```python
from build123d import *

# Parameters (mm, degrees)
SKETCH_1_R      = 25
EXTRUDE_1_DEPTH = 1
FILLET_1_R      = 1.6
EXTRUDE_START   = 5
EXTRUDE_3_DEPTH = 5
CHAMFER_3_SIZE  = 0.2


with BuildPart() as part:
    # 草图1 → 凸台-拉伸1 (new body)
    with BuildSketch(Plane.XY):
        Circle(SKETCH_1_R)
        with BuildLine():
            Line((-2.5, 1.658312395), (2.5, 1.658312395))
            ThreePointArc((2.5, 1.658312395), (0, -3), (-2.5, 1.658312395))
        make_face(mode=Mode.SUBTRACT)
        with BuildLine():
            ThreePointArc((-12.124355653, -7), (-7, -12.124355653), (0, -14))
            Line((0, -14), (0, -21))
            ThreePointArc((0, -21), (-10.5, -18.186533479), (-18.186533479, -10.5))
            Line((-18.186533479, -10.5), (-12.124355653, -7))
        make_face(mode=Mode.SUBTRACT)
        with BuildLine():
            ThreePointArc((0, 14), (-7, 12.124355653), (-12.124355653, 7))
            Line((-12.124355653, 7), (-18.186533479, 10.5))
            ThreePointArc((-18.186533479, 10.5), (-10.5, 18.186533479), (0, 21))
            Line((0, 21), (0, 14))
        make_face(mode=Mode.SUBTRACT)
        with BuildLine():
            Line((18.186533479, -10.5), (12.124355653, -7))
            ThreePointArc((12.124355653, -7), (14, 0), (12.124355653, 7))
            Line((12.124355653, 7), (18.186533479, 10.5))
            ThreePointArc((18.186533479, 10.5), (21, 0), (18.186533479, -10.5))
        make_face(mode=Mode.SUBTRACT)
    extrude(amount=-EXTRUDE_1_DEPTH)

    # 圆角1
    fillet_1_edges = [part.edges().sort_by_distance(p)[0] for p in [
        (-18.186533479, -10.5, -0.5),
        (0, -21, -0.5),
        (0, -14, -0.5),
        (-12.124355653, -7, -0.5),
        (18.186533479, -10.5, -0.5),
        (18.186533479, 10.5, -0.5),
        (12.124355653, 7, -0.5),
        (12.124355653, -7, -0.5),
        (-18.186533479, 10.5, -0.5),
        (-12.124355653, 7, -0.5),
        (0, 14, -0.5),
        (0, 21, -0.5),
    ]]
    fillet(fillet_1_edges, radius=FILLET_1_R)

    # 草图1<5> → 凸台-拉伸3 (add)
    with BuildSketch(Plane.XY.offset(EXTRUDE_START)):
        with BuildLine():
            ThreePointArc((-3, 0), (-2.598076211, 1.5), (-1.5, 2.598076211))
            Line((-1.5, 2.598076211), (-3, 5.196152423))
            ThreePointArc((-3, 5.196152423), (-5.196152423, 3), (-6, 0))
            Line((-6, 0), (-3, 0))
        make_face()
        with BuildLine():
            ThreePointArc((1.5, 2.598076211), (2.598076211, 1.5), (3, 0))
            Line((3, 0), (6, 0))
            ThreePointArc((6, 0), (5.196152423, 3), (3, 5.196152423))
            Line((3, 5.196152423), (1.5, 2.598076211))
        make_face()
        with BuildLine():
            ThreePointArc((1.5, -2.598076211), (0, -3), (-1.5, -2.598076211))
            Line((-1.5, -2.598076211), (-3, -5.196152423))
            ThreePointArc((-3, -5.196152423), (0, -6), (3, -5.196152423))
            Line((3, -5.196152423), (1.5, -2.598076211))
        make_face()
    extrude(amount=-EXTRUDE_3_DEPTH)

    # 倒角3
    chamfer_3_edges = [part.edges().sort_by_distance(p)[0] for p in [
        (-0.412026073, 14.44594919, -1),
        (-0.516287404, 20.511009142, -1),
        (0, 1.658312395, -1),
        (-4.5, 0, 5),
        (-2.598076211, 1.5, 5),
        (-2.25, 3.897114317, 5),
        (-5.196152423, 3, 5),
        (2.25, 3.897114317, 5),
        (2.598076211, 1.5, 5),
        (4.5, 0, 5),
        (5.196152423, 3, 5),
        (2.25, -3.897114317, 5),
        (0, -3, 5),
        (-2.25, -3.897114317, 5),
        (0, -6, 5),
        (-25, 0, -1),
        (-10.5, -18.186533479, -1),
        (-15.091202728, -8.712909958, -1),
        (-7, -12.124355653, -1),
        (0, -17.425819915, -1),
        (21, 0, -1),
        (15.091202728, -8.712909958, -1),
        (15.091202728, 8.712909958, -1),
        (14, 0, -1),
        (-15.091202728, 8.712909958, -1),
        (-10.5, 18.186533479, -1),
        (-7, 12.124355653, -1),
        (0, 17.425819915, -1),
        (-17.504911272, -10.702622579, -1),
        (0, -3, -1),
        (-12.304545944, -7.579799641, -1),
        (-0.412026073, -14.44594919, -1),
        (-0.516287404, -20.511009142, -1),
        (18.021198676, -9.808386563, -1),
        (18.021198676, 9.808386563, -1),
        (12.716572017, 6.866149549, -1),
        (12.716572017, -6.866149549, -1),
        (-17.504911272, 10.702622579, -1),
        (-12.304545944, 7.579799641, -1),
    ]]
    chamfer(chamfer_3_edges, length=CHAMFER_3_SIZE)


solid = part.part
```
Design review of the part built by this model. Coordinates are the model's own, in mm. A direction names the side the tool comes from. Give positions to 0.01 mm unless a question says otherwise; leave off trailing zeros. Write each loop counter-clockwise with the first axis right and the second up, starting at its lowest first coordinate (ties: lowest second). Pieces come first, ordered by that corner, then holes. Notation, with made-up numbers: (-32.5, 24) - (23.5, 24) arc R13 cw to (23.5, 39) - close; hole circle Ø9 at (30, 11.5). An arc over 180 degrees is marked (long way). Return JSON: item names as keys, results as strings. Group by question number.
(1) Mouldability with a two-part tool opening along Y and no side actions: class faces 1 (the flat face through (4, 0, 2)), 2 (the flat face through (-15.114, -8.726, -0.394)), 3 (the flat face through (4, 2, 5)) as +Y half, -Y half, draft (parallel to the pull), parting line (faces both ways), or undercut.
(2) We need section A-A, the plane z = 2. Give the boundary of the cut face in (x, y), then the cut area to 3 significant figures.
(3) Insertion check: pin 1 (8 mm diameter, centred on x = -4.5, y = -13.5, fed in from +Z); pin 2 (3 mm diameter, centred on y = -3.5, z = 2, fed in from +X); pin 3 (2 mm diameter, centred on y = 1, z = 2, fed in from +X); pin 4 (3 mm diameter, centred on y = 7, z = 3, fed in from -X). Each pin has a flat end and moves straight along its axis. Give the tip position at first contact, or say it passes through.
(4) To check wall thickness, follow probe 1 along Z at (x, y) = (7.5, 11); probe 2 along X at (y, z) = (12, -0.25); probe 3 along Y at (x, z) = (-4, 1). State the ranges of each line that lie inside material, in increasing order.
(5) Machinability: for faces 4 (the flat face through (0, -4, 5)), 5 (the cylindrical face through (0, -6, 2)), 6 (the flat face through (-15.07, 8.7, -0.39)), 7 (the flat face through (-2.24, -3.88, 2.43)), which of the approach directions +Z, -Z, +X, -X, +Y, -Y give a long, thin tool a straight path to every point of the face, cutting with its end or side? Answer none if there is none.
Reported:
{
 "1": {"face 1": "-Y half", "face 2": "undercut", "face 3": "draft"},
 "2": {"outline": "(-6, 0) - (-3, 0) arc R3 cw to (-1.5, 2.6) - (-3, 5.2) arc R6 ccw to start; (-3, -5.2) arc R6 ccw to (3, -5.2) - (1.5, -2.6) arc R3 cw to (-1.5, -2.6) - close; (1.5, 2.6) arc R3 cw to (3, 0) - (6, 0) arc R6 ccw to (3, 5.2) - close", "area": "42.4 mm2"},
 "3": {"pin 1": "stops at z = 0", "pin 2": "stops at x = 2.89", "pin 3": "stops at x = 6", "pin 4": "passes through"},
 "4": {"probe 1": "z = -1 to 0", "probe 2": "x = -21.93 to -17.23, -7.21 to 21.93", "probe 3": "y = 0 to 4.47"},
 "5": {"face 4": "+Z, +X, -X, +Y, -Y", "face 5": "+Z, -Y", "face 6": "+Z, -Z", "face 7": "+Z, -X"}
}
